Work out the finished part from the listing and answer in its coordinate system (mm). Round coordinates to 2 decimals unless told otherwise and drop trailing zeros. Loops run counter-clockwise (first coordinate to the right, second up) from the corner with the lowest first, then second, coordinate; pieces in that order, holes last. Notation, with made-up numbers: (-0.75, 84.25) - (43.25, 84.25) arc R37 ccw to (43.25, 120.25) - close; hole circle Ø6 at (-13, 10). An arc over 180 degrees is marked (long way). Return JSON: item names as keys, results as strings.
from build123d import *

# Parameters (mm, degrees)
SKETCH1_W      = 41.91
SKETCH1_H      = 2.54
EXTRUDE1_DEPTH = 2.54
SKETCH2_R      = 0.254
EXTRUDE2_DEPTH = 1.27
EXTRUDE4_START = 2.54
SKETCH3_R      = 0.254
EXTRUDE4_DEPTH = 2.54


with BuildPart() as part:
    # Sketch1 → Extrude1 (new body)
    with BuildSketch(Plane(origin=(0, 0, 0), x_dir=(1, 0, 0), z_dir=(0, 1, 0))):
        Rectangle(SKETCH1_W, SKETCH1_H)
    extrude(amount=EXTRUDE1_DEPTH)

    # Sketch2 → Extrude2 (add)
    with BuildSketch(Plane(origin=(0, 0, 0), x_dir=(1, 0, 0), z_dir=(0, 1, 0))):
        with Locations(Location((19.05, 0, 0), (0, 0, 270))):
            Circle(SKETCH2_R)
        with Locations(Location((16.51, 0, 0), (0, 0, 270))):
            Circle(SKETCH2_R)
        with Locations(Location((13.97, 0, 0), (0, 0, 270))):
            Circle(SKETCH2_R)
        with Locations(Location((11.43, 0, 0), (0, 0, 270))):
            Circle(SKETCH2_R)
        with Locations(Location((8.89, 0, 0), (0, 0, 270))):
            Circle(SKETCH2_R)
        with Locations(Location((6.35, 0, 0), (0, 0, 270))):
            Circle(SKETCH2_R)
        with Locations(Location((3.81, 0, 0), (0, 0, 270))):
            Circle(SKETCH2_R)
        with Locations(Location((1.27, 0, 0), (0, 0, 270))):
            Circle(SKETCH2_R)
        with Locations(Location((-1.27, 0, 0), (0, 0, 270))):
            Circle(SKETCH2_R)
        with Locations(Location((-3.81, 0, 0), (0, 0, 270))):
            Circle(SKETCH2_R)
        with Locations(Location((-6.35, 0, 0), (0, 0, 270))):
            Circle(SKETCH2_R)
        with Locations(Location((-8.89, 0, 0), (0, 0, 270))):
            Circle(SKETCH2_R)
        with Locations(Location((-11.43, 0, 0), (0, 0, 270))):
            Circle(SKETCH2_R)
        with Locations(Location((-13.97, 0, 0), (0, 0, 270))):
            Circle(SKETCH2_R)
        with Locations(Location((-16.51, 0, 0), (0, 0, 270))):
            Circle(SKETCH2_R)
        with Locations(Location((-19.05, 0, 0), (0, 0, 270))):
            Circle(SKETCH2_R)
    extrude(amount=-EXTRUDE2_DEPTH)

    # Sketch3 → Extrude4 (add)
    with BuildSketch(Plane(origin=(0, 2.54, 0), x_dir=(1, 0, 0), z_dir=(0, 1, 0)).offset(EXTRUDE4_START)):
        with Locations(Location((6.35, 0, 0), (0, 0, 270))):
            Circle(SKETCH3_R)
        with Locations(Location((8.89, 0, 0), (0, 0, 270))):
            Circle(SKETCH3_R)
        with Locations(Location((11.43, 0, 0), (0, 0, 270))):
            Circle(SKETCH3_R)
        with Locations(Location((13.97, 0, 0), (0, 0, 270))):
            Circle(SKETCH3_R)
        with Locations(Location((16.51, 0, 0), (0, 0, 270))):
            Circle(SKETCH3_R)
        with Locations(Location((19.05, 0, 0), (0, 0, 270))):
            Circle(SKETCH3_R)
        with Locations(Location((-13.97, 0, 0), (0, 0, 270))):
            Circle(SKETCH3_R)
        with Locations(Location((-11.43, 0, 0), (0, 0, 270))):
            Circle(SKETCH3_R)
        with Locations(Location((-8.89, 0, 0), (0, 0, 270))):
            Circle(SKETCH3_R)
        with Locations(Location((-6.35, 0, 0), (0, 0, 270))):
            Circle(SKETCH3_R)
        with Locations(Location((-3.81, 0, 0), (0, 0, 270))):
            Circle(SKETCH3_R)
        with Locations(Location((-1.27, 0, 0), (0, 0, 270))):
            Circle(SKETCH3_R)
        with Locations(Location((1.27, 0, 0), (0, 0, 270))):
            Circle(SKETCH3_R)
        with Locations(Location((3.81, 0, 0), (0, 0, 270))):
            Circle(SKETCH3_R)
        with Locations(Location((-19.05, 0, 0), (0, 0, 270))):
            Circle(SKETCH3_R)
        with Locations(Location((-16.51, 0, 0), (0, 0, 270))):
            Circle(SKETCH3_R)
    extrude(amount=-EXTRUDE4_DEPTH)


solid = part.part
1) Section B-B (x = 5) is taken. Give the vertices of the cut face in (y, z).
Verdict:
{"outline": "(0, -1.27) - (2.54, -1.27) - (2.54, 1.27) - (0, 1.27) - close"}
2) Section A-A (y = 4) is taken. Count the separate pieces of the cut face and the enclosed holes in it, and give its area (3 significant figures).
Verdict:
{"separate pieces": "16", "enclosed holes": "0", "area": "3.24 mm2"}
3) Section C-C (z = 0.6) is taken. Give the vertices of the cut face in (x, y) (3 decimals).
Verdict:
{"outline": "(-20.955, 0) - (20.955, 0) - (20.955, 2.54) - (-20.955, 2.54) - close"}
4) Find the intervals of material crossed by L1, parallel to Y at x = -2, z = 0.8, in increasing order.
Verdict:
{"L1": "y = 0 to 2.54"}
